Autodesk Inventor part; units mm, degrees
ref_plane "YZ Plane" through (0, 0, 0) normal (1, 0, 0) x (0, 1, 0)
ref_plane "XZ Plane" through (0, 0, 0) normal (0, 1, 0) x (-1, 0, 0)
ref_plane "XY Plane" through (0, 0, 0) normal (0, 0, 1) x (1, 0, 0)
sketch "Sketch1" plane through (0, 0, 0) normal (0, 0, 1) x (1, 0, 0)
  line L0 (0, 0) -> (-30, 0)
  line L1 (-30, 0) -> (-30, 20)
  line L2 (-30, 20) -> (0, 20)
  line L3 (0, 20) -> (0, 0)
  line L4 (0, 20) -> (-30, 20)
  line L5 (-30, 20) -> (-30, 55)
  line L6 (-30, 55) -> (0, 55)
  line L7 (0, 55) -> (0, 20)
  line L8 (-20, 15) -> (-10, 15) construction
  line L9 (-10, 15) -> (-10, 5) construction
  line L10 (-10, 5) -> (-20, 5) construction
  line L11 (-20, 5) -> (-20, 15) construction
  line L12 (-15, 15) -> (-15, 20) construction
  line L13 (-20, 10) -> (-30, 10) construction
  circle A0 centre (-20, 15) radius 2.6
  circle A1 centre (-10, 5) radius 2.6
  dimension "d0" = 30
  dimension "d1" = 20
  dimension "d2" = 30
  dimension "d3" = 35
  dimension "d4" = 10
  dimension "d5" = 10
  dimension "d6" = 5.2
  dimension "d8" = 5.2
extrude "Extrusion1" add sketch "Sketch1" along normal blind 14.75
sketch "Sketch2" plane through (0, 0, 14.75) normal (0, 0, 1) x (1, 0, 0)
  line L0 (0, 0) -> (0, 55)
  line L1 (0, 20) -> (-30, 20)
  line L2 (-30, 20) -> (-30, 25)
  line L3 (-30, 25) -> (0, 25)
  line L4 (0, 25) -> (0, 20)
  line L5 (-30, 0) -> (0, 0)
  line L6 (-30, 55) -> (-30, 0)
  point P0 (0, 25)
  dimension "d14" = 5
  dimension "d15" = 20
extrude "Extrusion2" add sketch "Sketch2" along normal blind 51 contours L1 L2 L3 L0
sketch "Sketch3" plane through (0, 0, 65.75) normal (0, 0, 1) x (1, 0, 0)
  line L0 (-30, 25) -> (0, 25)
  line L1 (0, 25) -> (0, 55)
  line L2 (0, 55) -> (-30, 55)
  line L3 (-30, 55) -> (-30, 25)
  line L4 (-30, 20) -> (0, 20)
  line L5 (0, 20) -> (0, 25)
  line L6 (0, 25) -> (-30, 25)
  line L7 (-30, 25) -> (-30, 20)
  line L8 (-30, 0) -> (0, 0)
  line L9 (0, 0) -> (0, 20)
  line L10 (0, 20) -> (-30, 20)
  line L11 (-30, 20) -> (-30, 0)
  point P0 (0, 25)
extrude "Extrusion3" add sketch "Sketch3" along normal blind 4 contours L3 L2 L1 L0 | L0 L5 L4 L7
sketch "Sketch4" plane through (0, 0, 0) normal (1, 0, 0) x (0, 0, -1)
  line L0 (-14.75, 55) -> (-14.75, 0)
  line L1 (-14.75, 20) -> (-6, 20)
  line L2 (-6, 20) -> (-6, 0)
  line L3 (-6, 0) -> (-14.75, 0)
  line L4 (-14.75, 0) -> (-14.75, 20)
  line L5 (0, 55) -> (-14.75, 55)
  line L6 (0, 55) -> (-10.75, 55)
  line L7 (-10.75, 55) -> (-10.75, 25)
  line L8 (-10.75, 25) -> (0, 25)
  line L9 (0, 25) -> (0, 55)
  line L10 (-14.75, 25) -> (-14.75, 55)
  line L11 (0, 0) -> (0, 55)
  point P0 (-14.75, 0)
  dimension "d21" = 20
  dimension "d22" = 30
  dimension "d23" = 4
  dimension "d50" = 6
extrude "Extrusion4" cut sketch "Sketch4" against normal through all
sketch "Sketch6" plane through (0, 0, 6) normal (0, 0, 1) x (1, 0, 0)
  line L0 (-30, 20) -> (0, 20)
  line L1 (-30, 0) -> (0, 0)
  line L2 (0, 20) -> (-4, 20)
  line L3 (-4, 20) -> (-4, 0)
  line L4 (-4, 0) -> (0, 0)
  line L5 (0, 0) -> (0, 20)
  line L6 (-30, 55) -> (-30, 20)
  line L7 (-30, 20) -> (-26, 20)
  line L8 (-26, 20) -> (-26, 0)
  line L9 (-26, 0) -> (-30, 0)
  line L10 (-30, 0) -> (-30, 20)
  point P0 (-26, 0)
  dimension "d33" = 4
  dimension "d34" = 4
extrude "Extrusion6" add sketch "Sketch6" along normal up to surface (63.75 mm away) contours L0 L8 L1 L10 | L0 L5 L1 L3
chamfer "Chamfer2" distance 63.75 distance2 20 1 edges at (-2, 0, 69.75) measured on face at (-1.3333, 0, 25.25)
chamfer "Chamfer3" distance 63.75 distance2 20 1 edges at (-28, 0, 69.75) measured on face at (-28.6667, 0, 25.25)
fillet "Fillet1" radius 15 4 edges at (-30, 55, 67.75) (0, 55, 67.75) (-30, 55, 12.75) (0, 55, 12.75)
sketch "Sketch7" plane through (0, 0, 69.75) normal (0, 0, 1) x (1, 0, 0)
  arc A0 (0, 40) -> (-30, 40) centre (-15, 40) ccw
  circle A1 centre (-15, 40) radius 3
  point P0 (0, 0)
  dimension "d44" = 6
extrude "Extrusion7" cut sketch "Sketch7" against normal through all
chamfer "Chamfer4" distance 3 angle 45 2 edges at (-18, 40, 14.75) (-18, 40, 65.75)
equation "\"d8\" = d6"
properties part number "X Axis Drag Chain Mount Moble"
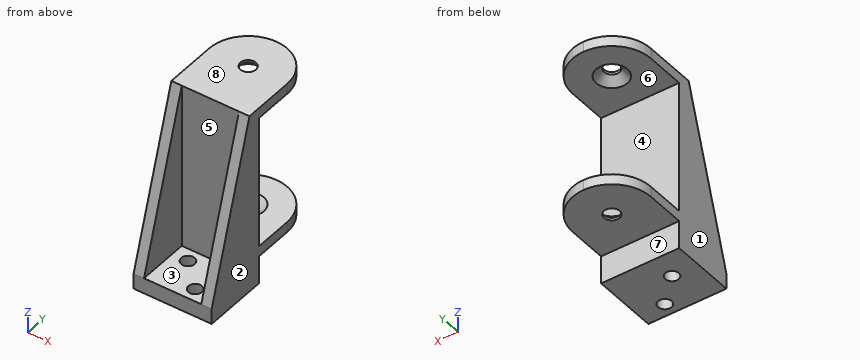
Build history of the part. All positions in model axes, mm. Face numbers are marked on the shaded views. A direction names the side the tool comes from. Give positions to 0.01 mm unless a question says otherwise; leave off trailing zeros. Order: outer loops, then holes, each group sorted by start corner. A loop starts at its lowest first (then second) coordinate and runs counter-clockwise, first axis right, second up. Notation, with made-up numbers: M 3,88.5 L 60,88.5 A22 cw 60,95.5 Z; hole C -1,23.5 d8. An arc over 180 degrees is marked long. Use one line per item in the form item = value.
1) Drop flat-ended pins along their axis: pin 1 (8.5 mm diameter, centred on x = -20, z = 4.5, fed in from +Y); pin 2 (7 mm diameter, centred on x = -20, y = 15, fed in from +Z); pin 3 (9 mm diameter, centred on x = -21, y = 47, fed in from -Z). Give the stop position or say it passes through.
Calculated:
pin_1 = 25
pin_2 = 6
pin_3 = 10.75
2) Saw through at A-A (y = 33). Give the cut face in (x, z).
Calculated:
outline = M -30,10.75 L 0,10.75 L 0,14.75 L -30,14.75 Z; M -30,65.75 L 0,65.75 L 0,69.75 L -30,69.75 Z
3) Tool access for the marked faces 5, 6, 7 and 8: list every direction of +Z, -Z, +X, -X, +Y, -Y with a clear straight run to the whole face (end or side of a thin tool).
Calculated:
face_5 = +Z, -Y
face_6 = +X, -X, +Y
face_7 = -Z, +X, -X, +Y
face_8 = +Z, +X, -X, +Y, -Y
4) Two-plate mould, pull along X, no slides. Class the marked faces 1, 2, 3 and 4: released by +X, released by -X, zero draft, split by the parting line, or undercut.
Calculated:
face_1 = released by -X
face_2 = released by +X
face_3 = undercut
face_4 = zero draft
5) Saw through at C-C (y = 50.5). Give the cut face in (x, z), plus the area to 3 significant figures.
Calculated:
outline = M -25.71,10.75 L -4.29,10.75 L -4.29,14.75 L -25.71,14.75 Z; M -25.71,65.75 L -4.29,65.75 L -4.29,69.75 L -25.71,69.75 Z
area = 171 mm2
6) Probe probe 1 along Y at (x, z) = (-15, 11); probe 2 along Y at (x, z) = (-20, 2.95); probe 3 along X at (y, z) = (5, 2.7). List the from-to ranges inside material, lowest first.
Calculated:
probe_1 = 20 to 37, 43 to 55
probe_2 = 0 to 12.4, 17.6 to 25
probe_3 = -30 to -12.6, -7.4 to 0
7) Saw through at B-B (x = -5). Give the cut face in (y, z).
Calculated:
outline = M 0,0 L 25,0 L 25,10.75 L 51.18,10.75 L 51.18,14.75 L 25,14.75 L 25,65.75 L 51.18,65.75 L 51.18,69.75 L 20,69.75 L 20,6 L 0,6 Z
